```python
from build123d import *

# Parameters (mm, degrees)
SKETCH1_R                = 2
BOSS_EXTRUDE1_DEPTH      = 4
BOSS_EXTRUDE2_DEPTH      = 6
CUT_EXTRUDE1_START       = -2
CUT_EXTRUDE1_DEPTH       = 18
SKETCH4_W                = 12.2
SKETCH4_H                = 11
CUT_EXTRUDE2_DEPTH       = 10
SKETCH5_W                = 20
SKETCH5_H                = 2
BOSS_EXTRUDE3_DEPTH      = 35
CUT_EXTRUDE7_DEPTH       = 112.736296699
SKETCH14_W               = 20
SKETCH14_H               = 2
CUT_EXTRUDE8_DEPTH       = 142.58036587
FILLET2_R                = 10
FILLET3_R                = 5
CUT_EXTRUDE10_DEPTH      = 142.58036587
CUT_EXTRUDE10_DEPTH_BACK = 142.58036587
SKETCH20_W               = 20
SKETCH20_H               = 4
BOSS_EXTRUDE5_DEPTH      = 2.5
CUT_EXTRUDE11_DEPTH      = 1
SKETCH26_W               = 13.25
SKETCH26_H               = 0.5
BOSS_EXTRUDE6_DEPTH      = 111
SKETCH31_R               = 2.75
SKETCH31_R_2             = 1.25
BOSS_EXTRUDE8_DEPTH      = 8
SKETCH31_5_R             = 2.75
SKETCH31_5_R_2           = 1.25
BOSS_EXTRUDE9_DEPTH      = 6
SKETCH33_R               = 1.25
CUT_EXTRUDE12_DEPTH      = 142.894547112
FILLET4_R                = 2
SKETCH34_W               = 103
SKETCH34_H               = 0.7
CUT_EXTRUDE13_DEPTH      = 2.4
CUT_EXTRUDE14_REACH      = 143.895
SKETCH35_W               = 27.5
SKETCH35_H               = 0.5
CUT_EXTRUDE15_REACH      = 145.183
SKETCH36_W               = 0.5
SKETCH36_H               = 3.5


with BuildPart() as part:
    # Sketch1 → Boss-Extrude1 (new, symmetric)
    with BuildSketch(Plane(origin=(0, 0, 0), x_dir=(1, 0, 0), z_dir=(0, 1, 0))):
        with BuildLine():
            ThreePointArc((-4, 7.5), (-11.5, 0), (-4, -7.5))
            Line((-4, -7.5), (0, -7.5))
            Line((0, -7.5), (0, 7.5))
            Line((0, 7.5), (-4, 7.5))
        make_face()
        with Locations(Location((-4, 0, 0), (0, 0, 270))):
            Circle(SKETCH1_R, mode=Mode.SUBTRACT)
    extrude(amount=BOSS_EXTRUDE1_DEPTH, both=True)

    # Sketch1<3> → Boss-Extrude2 (add, symmetric)
    with BuildSketch(Plane(origin=(0, 0, 0), x_dir=(1, 0, 0), z_dir=(0, 1, 0))):
        Polygon((0, 10), (0, 7.5), (0, 0), (141, 0), (141, 10), align=None)
        Polygon((0, 0), (0, -7.5), (0, -10), (141, -10), (141, 0), align=None)
    extrude(amount=BOSS_EXTRUDE2_DEPTH, both=True)

    # Sketch3 → Cut-Extrude1 (cut)
    with BuildSketch(Plane.ZY.offset(CUT_EXTRUDE1_START)):
        with BuildLine():
            Line((-3.494281042, -5), (3.494281042, -5))
            ThreePointArc((3.494281042, -5), (5.4094877, -2.819120931), (6.1, 0))
            Line((6.1, 0), (6.1, 6))
            Line((6.1, 6), (-6.1, 6))
            Line((-6.1, 6), (-6.1, 0))
            ThreePointArc((-6.1, 0), (-5.4094877, -2.819120931), (-3.494281042, -5))
        make_face()
    extrude(amount=-CUT_EXTRUDE1_DEPTH, mode=Mode.SUBTRACT)

    # Sketch4 → Cut-Extrude2 (cut)
    with BuildSketch(Plane.ZY.offset(-20)):
        with Locations((0, 0.5)):
            Rectangle(SKETCH4_W, SKETCH4_H)
    extrude(amount=-CUT_EXTRUDE2_DEPTH, mode=Mode.SUBTRACT)

    # Sketch5 → Boss-Extrude3 (add)
    with BuildSketch(Plane.ZY):
        with Locations((0, -7)):
            Rectangle(SKETCH5_W, SKETCH5_H)
    extrude(amount=-BOSS_EXTRUDE3_DEPTH)

    # Sketch13 → Cut-Extrude7 (cut, through all)
    with BuildSketch(Plane.ZY.offset(-30)):
        Polygon((-6.625, 5), (-6.625, -1), (-6.625, -5), (6.625, -5), (6.625, -1), (6.625, 5), align=None)
    extrude(amount=-CUT_EXTRUDE7_DEPTH, mode=Mode.SUBTRACT)

    # Sketch14 → Cut-Extrude8 (cut, through all)
    with BuildSketch(Plane.ZY):
        with Locations((0, 5)):
            Rectangle(SKETCH14_W, SKETCH14_H)
    extrude(amount=-CUT_EXTRUDE8_DEPTH, mode=Mode.SUBTRACT)

    # Fillet2
    # the kernel refuses this fillet: 10 mm, written as the material it adds along each edge
    with BuildSketch(Plane(origin=(35, -6, -10), x_dir=(1, 0, 0), z_dir=(0, 0, 1))) as fillet2_piece_1:
        with BuildLine():
            CenterArc((6, -10), FILLET2_R, 90, 36.869897646)
            Line((0, -2), (-0.12, -1.84))
            ThreePointArc((-0.12, -1.84), (-0.2, -1), (-0.2, 0))
            Line((-0.2, 0), (0, 0.2))
            Line((0, 0.2), (6, 0.2))
            Line((6, 0.2), (6, 0))
        make_face()
    extrude(amount=20)

    # Fillet3
    # the kernel refuses this fillet: 5 mm, written as the material it adds along each edge
    with BuildSketch(Plane(origin=(0, -4, 7.5), x_dir=(0, 0, 1), z_dir=(0, 1, 0))) as fillet3_piece_1:
        with BuildLine():
            CenterArc((4.995572165, -4.332680414), FILLET3_R, 119.941428639, 58.533496592)
            Line((-0.002656701, -4.199608248), (-0.502479587, -4.186301032))
            ThreePointArc((-0.502479587, -4.186301032), (-0.5, -4), (-0.5, 0))
            Line((-0.5, 0), (0, 0.5))
            ThreePointArc((0, 0.5), (1.25, 0.5), (2.250442783, 0.433268041))
            Line((2.250442783, 0.433268041), (2.5, 0))
        make_face()
    extrude(amount=8)
    with BuildSketch(Plane(origin=(0, -4, -7.5), x_dir=(0, 0, -1), z_dir=(0, 1, 0))) as fillet3_piece_2:
        with BuildLine():
            CenterArc((4.995572165, 4.332680414), FILLET3_R, 181.525074769, 58.533496592)
            Line((-0.002656701, 4.199608248), (-0.502479587, 4.186301032))
            ThreePointArc((-0.502479587, 4.186301032), (-0.5, 4), (-0.5, 0))
            Line((-0.5, 0), (0, -0.5))
            ThreePointArc((0, -0.5), (1.25, -0.5), (2.250442783, -0.433268041))
            Line((2.250442783, -0.433268041), (2.5, 0))
        make_face()
    extrude(amount=8)

    # Sketch20 → Cut-Extrude10 (cut, two sides: drawn at the far end of the back side and taken through both)
    with BuildSketch(Plane(origin=(0, 0, 0), x_dir=(0, 0, -1), z_dir=(1, 0, 0)).offset(-CUT_EXTRUDE10_DEPTH_BACK)):
        with Locations((0, 2)):
            Rectangle(SKETCH20_W, SKETCH20_H)
    extrude(amount=CUT_EXTRUDE10_DEPTH + CUT_EXTRUDE10_DEPTH_BACK, mode=Mode.SUBTRACT)

    # Sketch16 → Boss-Extrude5 (add)
    with BuildSketch(Plane(origin=(2, 0, 0), x_dir=(0, 0, -1), z_dir=(1, 0, 0))):
        with BuildLine():
            Line((-2.304886114, -1.5), (-5.9126982, -1.5))
            ThreePointArc((-5.9126982, -1.5), (-5.018497246, -3.467662813), (-3.494281042, -5))
            Line((-3.494281042, -5), (3.494281042, -5))
            ThreePointArc((3.494281042, -5), (5.018497246, -3.467662813), (5.9126982, -1.5))
            Line((5.9126982, -1.5), (2.304886114, -1.5))
            ThreePointArc((2.304886114, -1.5), (0, -2.75), (-2.304886114, -1.5))
        make_face()
    extrude(amount=BOSS_EXTRUDE5_DEPTH)

    # Sketch22 → Cut-Extrude11 (cut)
    with BuildSketch(Plane(origin=(0, 0, 0), x_dir=(1, 0, 0), z_dir=(0, 1, 0))):
        Polygon((2, 5.15), (2, 2.85), (-2.349469206, 7.905705794), (-1.064221101, 8.711768032), align=None)
        Polygon((2, -5.15), (2, -2.85), (-2.349469206, -7.905705794), (-1.064221101, -8.711768032), align=None)
    extrude(amount=-CUT_EXTRUDE11_DEPTH, mode=Mode.SUBTRACT)

    # Sketch26 → Boss-Extrude6 (add)
    with BuildSketch(Plane(origin=(141, 0, 0), x_dir=(0, 0, -1), z_dir=(1, 0, 0))):
        with Locations((0, -4.75)):
            Rectangle(SKETCH26_W, SKETCH26_H)
    extrude(amount=-BOSS_EXTRUDE6_DEPTH)

    # Sketch31 → Boss-Extrude8 (add, through all)
    # profile 1 of 2: a face of its own
    with BuildSketch(Plane(origin=(0, 0, 0), x_dir=(1, 0, 0), z_dir=(0, 1, 0))):
        with Locations((25, 11)):
            Circle(SKETCH31_R)
        with Locations((25, 11)):
            Circle(SKETCH31_R_2, mode=Mode.SUBTRACT)
    # profile 2 of 2: a face of its own
    with BuildSketch(Plane(origin=(0, 0, 0), x_dir=(1, 0, 0), z_dir=(0, 1, 0))):
        with Locations((25, -11)):
            Circle(SKETCH31_R)
        with Locations((25, -11)):
            Circle(SKETCH31_R_2, mode=Mode.SUBTRACT)
    extrude(amount=-BOSS_EXTRUDE8_DEPTH)

    # Sketch31<5> → Boss-Extrude9 (add)
    # profile 1 of 6: a face of its own
    with BuildSketch(Plane(origin=(0, 0, 0), x_dir=(1, 0, 0), z_dir=(0, 1, 0))):
        with Locations((25, 11)):
            Circle(SKETCH31_5_R)
        with Locations((25, 11)):
            Circle(SKETCH31_5_R_2, mode=Mode.SUBTRACT)
    # profile 2 of 6: a face of its own
    with BuildSketch(Plane(origin=(0, 0, 0), x_dir=(1, 0, 0), z_dir=(0, 1, 0))):
        with Locations((75, 11)):
            Circle(SKETCH31_5_R)
        with Locations((75, 11)):
            Circle(SKETCH31_5_R_2, mode=Mode.SUBTRACT)
    # profile 3 of 6: a face of its own
    with BuildSketch(Plane(origin=(0, 0, 0), x_dir=(1, 0, 0), z_dir=(0, 1, 0))):
        with Locations((125, 11)):
            Circle(SKETCH31_5_R)
        with Locations((125, 11)):
            Circle(SKETCH31_5_R_2, mode=Mode.SUBTRACT)
    # profile 4 of 6: a face of its own
    with BuildSketch(Plane(origin=(0, 0, 0), x_dir=(1, 0, 0), z_dir=(0, 1, 0))):
        with Locations((125, -11)):
            Circle(SKETCH31_5_R)
        with Locations((125, -11)):
            Circle(SKETCH31_5_R_2, mode=Mode.SUBTRACT)
    # profile 5 of 6: a face of its own
    with BuildSketch(Plane(origin=(0, 0, 0), x_dir=(1, 0, 0), z_dir=(0, 1, 0))):
        with Locations((75, -11)):
            Circle(SKETCH31_5_R)
        with Locations((75, -11)):
            Circle(SKETCH31_5_R_2, mode=Mode.SUBTRACT)
    # profile 6 of 6: a face of its own
    with BuildSketch(Plane(origin=(0, 0, 0), x_dir=(1, 0, 0), z_dir=(0, 1, 0))):
        with Locations((25, -11)):
            Circle(SKETCH31_5_R)
        with Locations((25, -11)):
            Circle(SKETCH31_5_R_2, mode=Mode.SUBTRACT)
    extrude(amount=-BOSS_EXTRUDE9_DEPTH)

    # Sketch33 → Cut-Extrude12 (cut, through all)
    with BuildSketch(Plane(origin=(0, 0, 0), x_dir=(1, 0, 0), z_dir=(0, 1, 0))):
        with Locations(Location((25, 11, 0), (0, 0, 270))):
            Circle(SKETCH33_R)
        with Locations(Location((75, 11, 0), (0, 0, 270))):
            Circle(SKETCH33_R)
        with Locations(Location((75, -11, 0), (0, 0, 270))):
            Circle(SKETCH33_R)
        with Locations(Location((25, -11, 0), (0, 0, 90))):
            Circle(SKETCH33_R)
        with Locations(Location((125, 11, 0), (0, 0, 270))):
            Circle(SKETCH33_R)
        with Locations(Location((125, -11, 0), (0, 0, 270))):
            Circle(SKETCH33_R)
    extrude(amount=-CUT_EXTRUDE12_DEPTH, mode=Mode.SUBTRACT)

    # Fillet4
    fillet4_edges = [part.edges().sort_by_distance(p)[0] for p in [
        (27.561737691, -4, 10),
        (22.438262309, -4, 10),
        (22.438262309, -4, -10),
        (27.561737691, -4, -10),
        (72.438262309, -3, -10),
        (77.561737691, -3, -10),
        (122.438262309, -3, -10),
        (127.561737691, -3, -10),
        (127.561737691, -3, 10),
        (122.438262309, -3, 10),
        (77.561737691, -3, 10),
        (72.438262309, -3, 10),
    ]]
    fillet(fillet4_edges, radius=FILLET4_R)

    # Sketch34 → Cut-Extrude13 (cut)
    with BuildSketch(Plane(origin=(0, 0, 0), x_dir=(1, 0, 0), z_dir=(0, 1, 0))):
        with Locations((81.5, 6.975)):
            Rectangle(SKETCH34_W, SKETCH34_H)
    cut_extrude13 = extrude(amount=-CUT_EXTRUDE13_DEPTH, mode=Mode.SUBTRACT)

    # Mirror1: Cut-Extrude13 across plane
    add(cut_extrude13.mirror(Plane.XY), mode=Mode.SUBTRACT)

    # Sketch35 → Cut-Extrude14 (cut, up to next)
    with BuildSketch(Plane.ZY, mode=Mode.PRIVATE) as cut_extrude14_sk1:
        with Locations((0, -7.75)):
            Rectangle(SKETCH35_W, SKETCH35_H)
    cut_extrude14_tool1 = extrude(cut_extrude14_sk1.sketch, amount=-CUT_EXTRUDE14_REACH, mode=Mode.PRIVATE) & part.part
    add(cut_extrude14_tool1.solids().sort_by_distance((0, -7.75, 0))[0], mode=Mode.SUBTRACT)

    # Sketch36 → Cut-Extrude15 (cut, up to next)
    with BuildSketch(Plane.XY.offset(10), mode=Mode.PRIVATE) as cut_extrude15_sk1:
        with Locations((0.25, -5.75)):
            Rectangle(SKETCH36_W, SKETCH36_H)
    cut_extrude15_tool1 = extrude(cut_extrude15_sk1.sketch, amount=-CUT_EXTRUDE15_REACH, mode=Mode.PRIVATE) & part.part
    add(cut_extrude15_tool1.solids().sort_by_distance((0.25, -5.75, 10))[0], mode=Mode.SUBTRACT)


solid = part.part
```
Geometry check sheet. Reference: the model listing, model coordinates, mm. A direction names the side the tool comes from. Give positions to 0.01 mm unless a question says otherwise; leave off trailing zeros. Write each loop counter-clockwise with the first axis right and the second up, starting at its lowest first coordinate (ties: lowest second). Pieces come first, ordered by that corner, then holes. Notation, with made-up numbers: (50, -7.5) - (109, -7.5) arc R23 ccw to (109, 12.5) - close; hole circle Ø11 at (74, 62.5). An arc over 180 degrees is marked (long way). Use a Markdown table: item, result.
Q1. Go/stop test with flat-tipped pins: P1, Ø3.5, axis at x = -4, z = 0, coming from the +Y side; P2, Ø0.7, axis at x = 90, y = -1.5, coming from the +Z side; P3, Ø4, axis at x = 25.5, y = -1.5, coming from the +Z side; P4, Ø4, axis at x = 40.5, y = -3.5, coming from the -Z side. Record where each tip stops, or that it passes through.
Computed:
| item | result |
|---|---|
| P1 | passes through |
| P2 | stops at z = 10 |
| P3 | stops at z = 13.75 |
| P4 | stops at z = -10 |
Q2. Section check A-A, the plane x = 25. Enter the section's corners in (y, z).
Computed:
| item | result |
|---|---|
| outline | (-7.5, -13.75) - (0, -13.75) - (0, -12.25) - (-7.5, -12.25) - close; (-7.5, -9.75) - (0, -9.75) - (0, -6.1) - (-5, -6.1) - (-5, 6.1) - (0, 6.1) - (0, 9.75) - (-7.5, 9.75) - close; (-7.5, 12.25) - (0, 12.25) - (0, 13.75) - (-7.5, 13.75) - close |
Q3. Thickness scan on L1, parallel to Z at x = 125, y = -1.65 (3 decimals); L2, parallel to Z at x = 125, y = -4.45 (3 decimals); L3, parallel to X at y = -3.25, z = 11. Record the ranges inside material, lowest first. Write a range as [from, to].
Computed:
| item | result |
|---|---|
| L1 | z = [-13.75, -12.25], [-9.75, -7.325], [7.325, 9.75], [12.25, 13.75] |
| L2 | z = [-13.75, -12.25], [-9.75, -6.625], [6.625, 9.75], [12.25, 13.75] |
| L3 | x = [22.09, 23.75], [26.25, 27.91], [72.09, 73.75], [76.25, 77.91], [122.09, 123.75], [126.25, 127.91] |
Q4. Section check C-C, the plane x = 82. Enter the section's corners in (y, z) (3 decimals), then the cut area to 3 significant figures.
Computed:
| item | result |
|---|---|
| outline | (-6, -10) - (0, -10) - (0, -7.325) - (-2.4, -7.325) - (-2.4, -6.625) - (-4.5, -6.625) - (-4.5, 6.625) - (-2.4, 6.625) - (-2.4, 7.325) - (0, 7.325) - (0, 10) - (-6, 10) - close |
| area | 57.0 mm² |
Q5. Draft check along Z on faces 1 (the face through (10, -4, -10)), 2 (the face through (81, -1, 7.325)), 3 (the face through (141, -5, 2)). Enter one of: pulls with the +Z half, pulls with the -Z half, needs draft (parallel to the pull), parting line crosses it, or undercut.
Computed:
| item | result |
|---|---|
| face 1 | pulls with the -Z half |
| face 2 | undercut |
| face 3 | needs draft |
Q6. Set-up check for faces 4 (the face through (-7, -4, 0)), 5 (the face through (10, -4, 10)), 6 (the face through (-0.14, -0.49, 5.34)), 7 (the face through (25.05, -3.7, -12.25)): record each of +Z, -Z, +X, -X, +Y, -Y from which the full face is reachable in a straight line by a thin tool's end or side.
Computed:
| item | result |
|---|---|
| face 4 | +Z, -Z, -X, -Y |
| face 5 | +Z, -X, +Y, -Y |
| face 6 | +Y |
| face 7 | +Y, -Y |
Q7. Section check B-B, the plane z = 0. Enter the section's corners in (x, y).
Computed:
| item | result |
|---|---|
| outline | (-11.5, -4) - (-6, -4) - (-6, 0) - (-11.5, 0) - close; (-2, -4) - (0.5, -4) - (0.5, -7.5) - (35.73, -7.5) arc R10 cw to (41, -6) - (141, -6) - (141, -4.5) - (30, -4.5) - (30, -5) - (4.5, -5) - (4.5, -2.75) - (2, -2.75) - (2, 0) - (-2, 0) - close |
